Model file for the job. Use its own axes, mm. A direction names the side the tool comes from. Coordinates: 2 decimals unless noted, no trailing zeros. Order: outer loops, then holes, each group sorted by start corner. A loop starts at its lowest first (then second) coordinate and runs counter-clockwise, first axis right, second up.
Autodesk Fusion 360 part; units mm, degrees
sketch "Esboço1" plane through (0, 0, 0) normal (0, 0, 1) x (1, 0, 0)
  line L0 (-100, 200) -> (-100, 150)
  line L1 (-99.9888, 86.3572) -> (-99.9888, 36.3572)
  line L2 (-99.9888, 36.3572) -> (50.0112, 36.3572)
  line L3 (-100, 200) -> (50, 200)
  line L4 (50, 200) -> (50, 150)
  line L5 (50.0112, 36.3572) -> (50.0112, 86.3572)
  line L6 (-99.9888, 86.3572) -> (-85.8446, 100.4973)
  line L7 (50.0112, 86.3572) -> (35.8252, 100.4553)
  line L8 (50, 150) -> (35.8579, 135.8579)
  line L9 (-100, 150) -> (-85.8579, 135.8579)
  spline S0 degree 2 poles (-85.8446, 100.4973) (-80, 120) (-85.8579, 135.8579) knots 0 0 0 3.643978 3.643978 3.643978 weights 1 3 1
  spline S1 degree 2 poles (35.8252, 100.4553) (30, 120) (35.8579, 135.8579) knots 0 0 0 3.647748 3.647748 3.647748 weights 1 3 1
  dimension "d1" = 50
  dimension "d5" = 50
  dimension "d6" = 150
  dimension "d7" = 150
  dimension "d8" = 50
  dimension "d9" = 50
  dimension "d13" = 20
  dimension "d14" = 20
  dimension "d15" = 20
  dimension "d16" = 20
extrude "Extrusão1" add sketch "Esboço1" along normal blind 20
hole "Furo1" at (40, 190, 20) direction (0, 0, -1) diameter 2.5 depth 30 tip angle 118
hole "Furo2" at (40, 162.5, 20) direction (0, 0, -1) diameter 2.5 depth 30 tip angle 118
hole "Furo3" at (-90, 190, 20) direction (0, 0, -1) diameter 2.5 depth 30 tip angle 118
hole "Furo4" at (-90, 162.5, 20) direction (0, 0, -1) diameter 2.5 depth 30 tip angle 118
hole "Furo5" at (-89.9888, 73.8572, 20) direction (0, 0, -1) diameter 2.5 depth 30 tip angle 118
hole "Furo6" at (-89.9888, 46.3572, 20) direction (0, 0, -1) diameter 2.5 depth 30 tip angle 118
hole "Furo7" at (40.0112, 73.8572, 20) direction (0, 0, -1) diameter 2.5 depth 30 tip angle 118
hole "Furo8" at (40.0112, 46.3572, 20) direction (0, 0, -1) diameter 2.5 depth 30 tip angle 118
hole "Furo9" at (-42.4888, 48.3572, 20) direction (0, 0, -1) diameter 4 depth 30 tip angle 118
hole "Furo10" at (-7.4888, 48.3572, 20) direction (0, 0, -1) diameter 4 depth 30 tip angle 118
hole "Furo11" at (14.0112, 70.3572, 20) direction (0, 0, -1) diameter 3.5 depth 30 tip angle 118
hole "Furo12" at (-4.4888, 70.3572, 20) direction (0, 0, -1) diameter 3.5 depth 30 tip angle 118
hole "Furo13" at (-45.4888, 70.3572, 20) direction (0, 0, -1) diameter 3.5 depth 30 tip angle 118
hole "Furo14" at (-63.9888, 70.3572, 20) direction (0, 0, -1) diameter 3.5 depth 30 tip angle 118
Q1. Mould opens along X. For faces 1 (the face through (-26, 200, 10)), 2 (the face through (-7.577, 50.355, 9.86)), 3 (the face through (-93.016, 93.328, 9.86)), 4 (the face through (50.011, 61, 10)) say: pulls with the +X half, pulls with the -X half, needs draft (parallel to the pull), parting line crosses it, or undercut.
Established:
face 1: needs draft
face 2: undercut
face 3: pulls with the -X half
face 4: pulls with the +X half
Q2. Cut at B-B, the plane y = 139. List the corners of the cut face in (x, z), plus the area to 3 significant figures.
Established:
outline: (-89, 0) - (39, 0) - (39, 20) - (-89, 20) - close
area: 2,560 mm2
Q3. Cut at A-A, the plane z = 17. Count the separate pieces of the cut face and the enclosed holes in it, plus the area to 3 significant figures.
Established:
separate pieces: 1
enclosed holes: 14
area: 22,900 mm2
Q4. Which spindle directions (+Z, -Z, +X, -X, +Y, -Y) get a long thin tool onto all of the face, cutting with end or side? Do faces 5 (the face through (43.018, 93.308, 9.86)), 6 (the face through (-64.066, 72.106, 9.86)), 7 (the face through (-93, 143, 10)). Say none if no direction does.
Established:
face 5: +Z, -Z, +X
face 6: +Z, -Z
face 7: +Z, -Z, -X
Q5. Drop flat-ended pins along their axis: P1, Ø6.5, axis at x = -42.49, y = 48.36, coming from the -Z side; P2, Ø1.5, axis at y = 143.5, z = 14.5, coming from the -X side; P3, Ø6, axis at y = 174, z = 9.5, coming from the +X side; P4, Ø5, axis at y = 100.5, z = 5.5, coming from the +X side. Give the stop position or say it passes through.
Established:
P1: stops at z = 0
P2: stops at x = -94.25
P3: stops at x = 50
P4: stops at x = 38.3
Q6. Probe line 1 (Y direction, x = -90.5, z = 19); line 2 (X direction, y = 70, z = 9.75); line 3 (X direction, y = 71.5, z = 2.75). List the from-to ranges inside material, lowest first.
Established:
line 1: y = 36.36 to 45.22, 47.5 to 72.72, 75 to 95.84, 140.5 to 161.35, 163.65 to 188.85, 191.15 to 200
line 2: x = -99.99 to -65.7, -62.28 to -47.2, -43.78 to -6.2, -2.78 to 12.3, 15.72 to 50.01
line 3: x = -99.99 to -65.31, -62.66 to -46.81, -44.16 to -5.81, -3.16 to 12.69, 15.34 to 50.01
